Verification items for the finished model (mm, model axes). Give positions to 0.01 mm unless a question says otherwise; leave off trailing zeros. Order: outer loops, then holes, each group sorted by start corner. A loop starts at its lowest first (then second) coordinate and runs counter-clockwise, first axis right, second up.
(1) Sectioned sample at A-A on z = -19. Record the cut outline in (x, y), plus the area to 3 significant figures.
(2) Scan lines: L1, parallel to Y at x = -128.55, z = 3; L2, parallel to Z at x = -128.6, y = 110.8; L3, parallel to Z at x = -129.3, y = 163. Record each from-to range of solid material in increasing order.
(3) Sectioned sample at C-C on z = -1. Record the cut outline in (x, y).
(4) Mould release check, pull along Z, two halves, no side actions. Record for faces 1 (the face through (-128.48, 161.52, 3.17)), 2 (the face through (-129, 104, -9)), 3 (the face through (-129, 139, -29)): pulls with the +Z half, pulls with the -Z half, needs draft (parallel to the pull), parting line crosses it, or undercut.
(5) Gauge pin test, flat end, axial feed: pin 1 (1.4 mm diameter, centred on y = 114.3, z = -1, fed in from +X). Record the tip position at first contact, or that the pin passes through.
(6) Sectioned sample at B-B on y = 164. Record the cut outline in (x, z).
(7) Sectioned sample at D-D on z = 3. Record the cut outline in (x, y), plus the area to 3 significant figures.
```python
from build123d import *

# Parameters (mm, degrees)
SKETCH001_W             = 40
SKETCH001_H             = 70
PAD001_DEPTH            = 3
SKETCH002_R             = 2.25
HOLE_DEPTH              = 3.001
SKETCH003_R             = 0.8
HOLE001_DEPTH           = 3.001
BODY001_PLACEMENT_ANGLE = 90


with BuildPart() as part:
    # Sketch001 → Pad001 (new body)
    with BuildSketch(Plane.XY):
        Rectangle(SKETCH001_W, SKETCH001_H)
    extrude(amount=PAD001_DEPTH)

    # Sketch002 (on Face6 of Pad001) → Hole (cut, through all)
    with BuildSketch(Plane.XY.offset(3)):
        with Locations((10, 25)):
            Circle(SKETCH002_R)
        with Locations((10, -25)):
            Circle(SKETCH002_R)
    extrude(amount=-HOLE_DEPTH, mode=Mode.SUBTRACT)

    # Sketch003 (on Face5 of Hole) → Hole001 (cut, through all)
    with BuildSketch(Plane.XY.offset(3)):
        with Locations((-12, 23.3)):
            Circle(SKETCH003_R)
        with Locations((-12, -28.2)):
            Circle(SKETCH003_R)
        with Locations((-8, -24.7)):
            Circle(SKETCH003_R)
    extrude(amount=-HOLE001_DEPTH, mode=Mode.SUBTRACT)


with BuildPart() as part_1:
    # Body001 placement: moved
    add(part.part.moved(Location((-130, 139, -9))).rotate(Axis((-130, 139, -9), (0, 1, 0)), BODY001_PLACEMENT_ANGLE))


solid = part_1.part
```
Ans:
1. outline: (-130, 104) - (-127, 104) - (-127, 111.75) - (-130, 111.75) - close; (-130, 116.25) - (-127, 116.25) - (-127, 161.75) - (-130, 161.75) - close; (-130, 166.25) - (-127, 166.25) - (-127, 174) - (-130, 174) - close
1. area: 183 mm2
2. L1: y = 104 to 110, 111.6 to 161.5, 163.1 to 174
2. L2: z = -29 to 2.2, 3.8 to 11
2. L3: z = -29 to -21.02, -16.98 to 2.61, 3.39 to 11
3. outline: (-130, 104) - (-127, 104) - (-127, 113.5) - (-130, 113.5) - close; (-130, 115.1) - (-127, 115.1) - (-127, 174) - (-130, 174) - close
4. face 1: undercut
4. face 2: needs draft
4. face 3: pulls with the -Z half
5. pin 1: passes through
6. outline: (-130, -29) - (-127, -29) - (-127, -21.25) - (-130, -21.25) - close; (-130, -16.75) - (-127, -16.75) - (-127, 11) - (-130, 11) - close
7. outline: (-130, 104) - (-127, 104) - (-127, 110) - (-130, 110) - close; (-130, 111.6) - (-127, 111.6) - (-127, 161.5) - (-130, 161.5) - close; (-130, 163.1) - (-127, 163.1) - (-127, 174) - (-130, 174) - close
7. area: 200 mm2
